Part model, mm, in its own coordinate system. Face numbers are marked on the shaded views. Give positions to 0.01 mm unless a question says otherwise; leave off trailing zeros. Answer as CSV lines item,"result". Start each with the question number.
1) Pin check, flat tips, straight feed: pin 1 Ø4 at (y, z) = (68, -187.5) entering from -X; pin 2 Ø10 at (y, z) = (22.5, -52.5) entering from +X. Stop position of each tip, or through.
2) Wall check: line 1 along X through (y, z) = (52, -73); line 2 along X through (y, z) = (23, -61); line 3 along X through (y, z) = (35.5, -260.5). Give the ranges that are in metal, low to high. Write a range as from..to.
3) Mould opens along X. For the marked faces 1, 2 and 3 say: pulls with the +X half, pulls with the -X half, needs draft (parallel to the pull), parting line crosses it, or undercut.
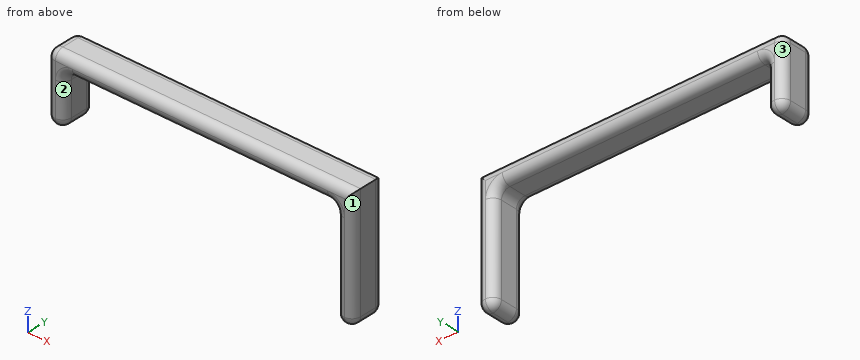
```python
from build123d import *

# Parameters (mm, degrees)
SKETCH1_W           = 812.8
SKETCH1_H           = 101.6
BOSS_EXTRUDE1_DEPTH = 50.8
SKETCH2_W           = 50.8
SKETCH2_H           = 101.6
BOSS_EXTRUDE2_DEPTH = 203.2
SKETCH6_W           = 365.887
SKETCH6_H           = 101.6
BOSS_EXTRUDE4_DEPTH = 50.8
FILLET2_R           = 25.4


with BuildPart() as part:
    # Sketch1 → Boss-Extrude1 (new body)
    with BuildSketch(Plane.XY):
        with Locations((-406.4, 50.8)):
            Rectangle(SKETCH1_W, SKETCH1_H)
    extrude(amount=BOSS_EXTRUDE1_DEPTH)

    # Sketch2 → Boss-Extrude2 (add)
    with BuildSketch(Plane.XY.offset(50.8)):
        with Locations((-838.2, 50.8)):
            Rectangle(SKETCH2_W, SKETCH2_H)
        with Locations((25.4, 50.8)):
            Rectangle(SKETCH2_W, SKETCH2_H)
    extrude(amount=-BOSS_EXTRUDE2_DEPTH)

    # Sketch6 → Boss-Extrude4 (add)
    with BuildSketch(Plane(origin=(50.8, 0, 0), x_dir=(0, 0, -1), z_dir=(1, 0, 0))):
        with Locations((132.1435, 50.8)):
            Rectangle(SKETCH6_W, SKETCH6_H)
    extrude(amount=-BOSS_EXTRUDE4_DEPTH)

    # Fillet2
    fillet2_edges = [part.edges().sort_by_distance(p)[0] for p in [
        (-406.4, 0, 50.8),
        (-812.8, 101.6, -76.2),
        (-812.8, 50.8, -152.4),
        (-838.2, 0, -152.4),
        (-812.8, 0, -76.2),
        (-863.6, 50.8, -152.4),
        (-863.6, 0, -50.8),
        (-838.2, 101.6, -152.4),
        (-863.6, 101.6, -50.8),
        (-863.6, 50.8, 50.8),
        (0, 0, -157.5435),
        (0, 101.6, -157.5435),
        (50.8, 101.6, -132.1435),
        (50.8, 0, -132.1435),
        (50.8, 50.8, -315.087),
        (25.4, 0, -315.087),
        (0, 50.8, -315.087),
        (25.4, 101.6, -315.087),
        (-406.4, 0, 0),
        (-812.8, 50.8, 0),
        (-406.4, 101.6, 0),
        (0, 50.8, 0),
        (-406.4, 101.6, 50.8),
    ]]
    fillet(fillet2_edges, radius=FILLET2_R - 0.0001)  # a hair under: the kernel refuses the full size


solid = part.part
```
Found:
1,pin 1,"x = 0"
1,pin 2,"x = 50.8"
2,line 1,"-863.6..-812.8, 0..50.8"
2,line 2,"-863.49..-812.91, 0.11..50.69"
2,line 3,"0..50.8"
3,face 1,"pulls with the +X half"
3,face 2,"undercut"
3,face 3,"pulls with the -X half"
